Design review of the part built by this model. Coordinates are the model's own, in mm. A direction names the side the tool comes from. Coordinates: 2 decimals unless noted, no trailing zeros. Loops run counter-clockwise (first coordinate to the right, second up) from the corner with the lowest first, then second, coordinate; pieces in that order, holes last. Notation, with made-up numbers: (-3, 57) -> (26, 57) arc R27 ccw to (26, 86) -> close; hole circle Ø3 at (19, -24). An arc over 180 degrees is marked (long way). Answer as a JSON object with one key per item and string values.
Autodesk Inventor part; units mm, degrees
ref_plane "XZ Plane" through (0, 0, 0) normal (0, 1, 0) x (-1, 0, 0)
ref_plane "XY Plane" through (0, 0, 0) normal (0, 0, 1) x (1, 0, 0)
sketch "Sketch1" plane through (0, 0, 0) normal (0, 0, 1) x (1, 0, 0)
  line L0 (0, 20.0573) -> (0, -21.2213)
  line L1 (0, -21.2213) -> (-7.3, -21.2213)
  line L2 (-7.3, -21.2213) -> (-7.3, -12.5213)
  line L3 (-7.3, -12.5213) -> (-10.65, -12.5213)
  line L4 (-10.65, 1.9287) -> (-12.425, 1.9287)
  line L5 (-12.425, 1.9287) -> (-12.425, 3.9287)
  line L6 (-12.425, 3.9287) -> (-10.1, 3.9287)
  line L7 (-10.1, 3.9287) -> (-10.1, 8.4287)
  line L8 (-10.1, 8.4287) -> (-12.5, 8.4287)
  line L9 (-12.5, 8.4287) -> (-12.5, 10.4287)
  line L10 (-12.5, 10.4287) -> (-15.9, 13.3766)
  line L11 (-15.9, 13.3766) -> (-15.9, 18.6266)
  line L12 (0, 23.9493) -> (0, -31.6262)
  line L13 (-10.65, -12.5213) -> (-10.65, 1.9287)
  line L14 (-15.9, 18.6266) -> (-7.775, 20.0573)
  line L15 (-7.775, 20.0573) -> (0, 20.0573)
  point P0 (0, 0)
  point P1 (-10.1, 6.1787)
  point P2 (-10.65, -5.2963)
  dimension "d2" = 31.8
  dimension "d3" = 25
  dimension "d5" = 20.2
  dimension "d6" = 24.85
  dimension "d9" = 14.6
  dimension "d10" = 8.7
  dimension "d13" = 2
  dimension "d14" = 4.5
  dimension "d15" = 4.5
  dimension "d16" = 2
  dimension "d17" = 5.25
  dimension "d19" = 21.3
  dimension "d20" = 14.45
  dimension "d21" = 15.55
  dimension "d22" = 8.25
revolve "Revolution1" add sketch "Sketch1" angle 360 about axis through (0, 23.9493, 0) along (0, -1, 0)
sketch "Sketch2" plane through (0, -21.2213, 0) normal (0, -1, 0) x (1, 0, 0)
  line L0 (6.6, 2.8) -> (3.6, 2.8)
  line L1 (3.6, 2.8) -> (3.6, 2.3)
  line L2 (3.6, 2.3) -> (6.6, 2.3)
  line L3 (6.6, 2.3) -> (6.6, 2.8)
  line L4 (1.5, 2.8) -> (-1.5, 2.8)
  line L5 (-1.5, 2.8) -> (-1.5, 2.3)
  line L6 (-1.5, 2.3) -> (1.5, 2.3)
  line L7 (1.5, 2.3) -> (1.5, 2.8)
  line L8 (-3.6, 2.8) -> (-6.6, 2.8)
  line L9 (-6.6, 2.8) -> (-6.6, 2.3)
  line L10 (-6.6, 2.3) -> (-3.6, 2.3)
  line L11 (-3.6, 2.3) -> (-3.6, 2.8)
  circle A0 centre (0, 0) radius 7.3
  point P0 (0, 0)
  dimension "d23" = 0.5
  dimension "d24" = 3
  dimension "d25" = 2.1
  dimension "d26" = 2.1
  dimension "d29" = 14.6
  dimension "d31" = 2.8
  dimension "d32" = 1.5
extrude "Extrusion1" add sketch "Sketch2" along normal blind 8 contours L3 L2 L1 L0 | L7 L6 L5 L4 | L11 L10 L9 L8
fillet "Fillet1" radius 1 6 edges at (6.6, -29.2213, 2.55) (3.6, -29.2213, 2.55) (-6.6, -29.2213, 2.55) (-3.6, -29.2213, 2.55) (-1.5, -29.2213, 2.55) (1.5, -29.2213, 2.55)
ref_plane "Work Plane1" through (6, 0, 0) normal (1, 0, 0) x (0, 1, 0)
sketch "Sketch3" plane through (6, 0, 0) normal (1, 0, 0) x (0, 1, 0)
  line L0 (-12.5213, 7.3) -> (-12.5213, -7.3)
  line L1 (-12.5213, 2.25) -> (-18.0213, 2.25)
  line L2 (-18.0213, 2.25) -> (-18.0213, -2.25)
  line L3 (-18.0213, -2.25) -> (-12.5213, -2.25)
  line L4 (-12.5213, -2.25) -> (-12.5213, 2.25)
  line L5 (-39.077, 0) -> (29.913, 0)
  point P0 (0, 0)
  dimension "d37" = 4.5
  dimension "d38" = 5.5
  dimension "d39" = 2.25
extrude "Extrusion2" add sketch "Sketch3" along normal blind 1.5
sketch "Sketch4" plane through (7.5, 0, 0) normal (1, 0, 0) x (0, 0, -1)
  line L0 (-2.25, -18.0213) -> (2.25, -18.0213)
  line L1 (-1.25, -15.5213) -> (1.25, -15.5213)
  line L2 (1.25, -15.5213) -> (1.25, -18.0213)
  line L3 (1.25, -18.0213) -> (-1.25, -18.0213)
  line L4 (-1.25, -18.0213) -> (-1.25, -15.5213)
  line L5 (0, -39.077) -> (0, 29.913)
  point P0 (0, 0)
  dimension "d42" = 2.5
  dimension "d43" = 2.5
  dimension "d44" = 1.25
extrude "Extrusion3" add sketch "Sketch4" along normal blind 1.6
equation "\"d39\" = 0.5 * d37"
equation "\"d44\" = 0.5 * d43"
properties part number "Co-1-01-eStopButton"
1) For faces 1 (the flat face through (5, -25, 2.3)), 2 (the flat face through (9.1, -17, 0)), 3 (the flat face through (0, -25, 2.8)), 4 (the flat face through (8, -15.521, 0)), list the 3-axis set-ups (+Z, -Z, +X, -X, +Y, -Y) from which the entire face can be reached by the end or side of a thin tool; tool diameter is ignored.
Completed:
{"face 1": "-Z, +X, -X, -Y", "face 2": "+Z, -Z, +X, -Y", "face 3": "+Z, +X, -X, -Y", "face 4": "+Z, -Z, +X"}
2) Add section B-B, the plane y = -6.5. Give the boundary of the cut face in (x, z).
Completed:
{"outline": "circle Ø21.3 at (0, 0)"}
3) Clearance check with flat-ended pins moving along their axes: pin 1 Ø0.6 at (y, z) = (-26.5, 2.5) entering from +X; pin 2 Ø6 at (x, y) = (3.5, -18.5) entering from -Z; pin 3 Ø0.6 at (x, y) = (7.5, -15.5) entering from -Z. State where each tip first meets the part, or that it passes through.
Completed:
{"pin 1": "x = 6.6", "pin 2": "z = -7.28", "pin 3": "z = -2.25"}
4) Wall thickness on probe 1 along Y at (x, z) = (4, -11); probe 2 along Y at (x, z) = (5, -3.5); probe 3 along Z at (x, y) = (0, -4.5): over which ranges is each line inside the solid? List them lowest first.
Completed:
{"probe 1": "1.93 to 3.93, 8.43 to 19.37", "probe 2": "-21.22 to 20.06", "probe 3": "-10.65 to 10.65"}
5) Add section C-C, the plane y = 17. Give the boundary of the cut face in (x, z).
Completed:
{"outline": "circle Ø31.8 at (0, 0)"}
